Input: part model. Units: mm. Frame: model coordinates. Coordinates: 2 decimals unless noted, no trailing zeros. Use a Markdown table: item, result. Add a question column.
1. Section A-A on x = 4. State how many separate pieces and enclosed holes the cut face has, then the cut area to 3 significant figures.
2. Draft query along Y for faces 1 (the flat face through (4.31, 2.63, -33.57)), 2 (the flat face through (4, 10, -9)), 3 (the cylindrical face through (4.19, 5.676, -7.146)), 4 (the cylindrical face through (4.19, 5.676, -29.146)). Return one class per face: +Y half, -Y half, draft (parallel to the pull), parting line (faces both ways), or undercut.
3. Line query: L1, parallel to Z at x = 1.5, y = 3; L2, parallel to Z at x = 4.5, y = 7; L3, parallel to Y at x = 6.5, z = -5. Output: solid intervals per line, ascending. Write a range as [from, to].
4. Pin query (flat end, axial travel): pin 1 (3.5 mm diameter, centred on y = 5, z = -5, fed in from -X); pin 2 (1 mm diameter, centred on x = 6, y = 8, fed in from +Z); pin 3 (1 mm diameter, centred on x = 1.5, z = -30.5, fed in from -Y); pin 4 (1.5 mm diameter, centred on x = 1.5, y = 3, fed in from +Z). Return the tip coordinate at first contact, or that it passes through.
```python
from build123d import *

# Parameters (mm, degrees)
SKETCH1_R           = 2.25
BOSS_EXTRUDE1_DEPTH = 8.5
BOSS_EXTRUDE2_DEPTH = 8.5


with BuildPart() as part:
    # Sketch1 → Boss-Extrude1 (new body)
    with BuildSketch(Plane(origin=(0, 0, 0), x_dir=(0, 0, -1), z_dir=(1, 0, 0))):
        with BuildLine():
            Line((27, 10), (5, 10))
            ThreePointArc((5, 10), (0, 5), (5, 0))
            Line((5, 0), (27, 0))
            ThreePointArc((27, 0), (32, 5), (27, 10))
        make_face()
        with Locations((5, 5)):
            Circle(SKETCH1_R, mode=Mode.SUBTRACT)
        with Locations((27, 5)):
            Circle(SKETCH1_R, mode=Mode.SUBTRACT)
    extrude(amount=BOSS_EXTRUDE1_DEPTH)

    # Sketch2 → Boss-Extrude2 (add)
    with BuildSketch(Plane(origin=(8.5, 0, 0), x_dir=(0, 0, -1), z_dir=(1, 0, 0))):
        with BuildLine():
            add(Edge.make_bspline(
                [(63.752972286, 17.872423117), (45.928882678, 26.563787963), (31.059268621, 10), (13.694974759, 10)],
                knots=[0, 0, 0, 0, 1, 1, 1, 1], degree=3))
            Line((13.694974759, 10), (27, 10))
            ThreePointArc((27, 10), (31.87285141, 6.120410255), (29.183837075, 0.502127655))
            Line((29.183837075, 0.502127655), (38.08542066, 4.824084077))
            add(Edge.make_bspline(
                [(38.08542066, 4.824084077), (46.797509509, 11.895222457), (57.948000409, 11.067843667)],
                knots=[0, 0, 0, 1, 1, 1], degree=2))
            Line((57.948000409, 11.067843667), (65.313809691, 14.189518476))
            Line((65.313809691, 14.189518476), (63.752972286, 17.872423117))
        make_face()
    extrude(amount=-BOSS_EXTRUDE2_DEPTH)


solid = part.part
```
Answers below:
| question | item | result |
|---|---|---|
| 1 | separate pieces | 1 |
| 1 | enclosed holes | 2 |
| 1 | area | 622 mm² |
| 2 | face 1 | -Y half |
| 2 | face 2 | +Y half |
| 2 | face 3 | undercut |
| 2 | face 4 | undercut |
| 3 | L1 | z = [-34.33, -28.03], [-25.97, -6.03], [-3.97, -0.42] |
| 3 | L2 | z = [-41.12, -28.03], [-25.97, -6.03], [-3.97, -0.42] |
| 3 | L3 | y = [0, 2.75], [7.25, 10] |
| 4 | pin 1 | passes through |
| 4 | pin 2 | stops at z = -0.67 |
| 4 | pin 3 | stops at y = 0.9 |
| 4 | pin 4 | stops at z = -0.16 |
